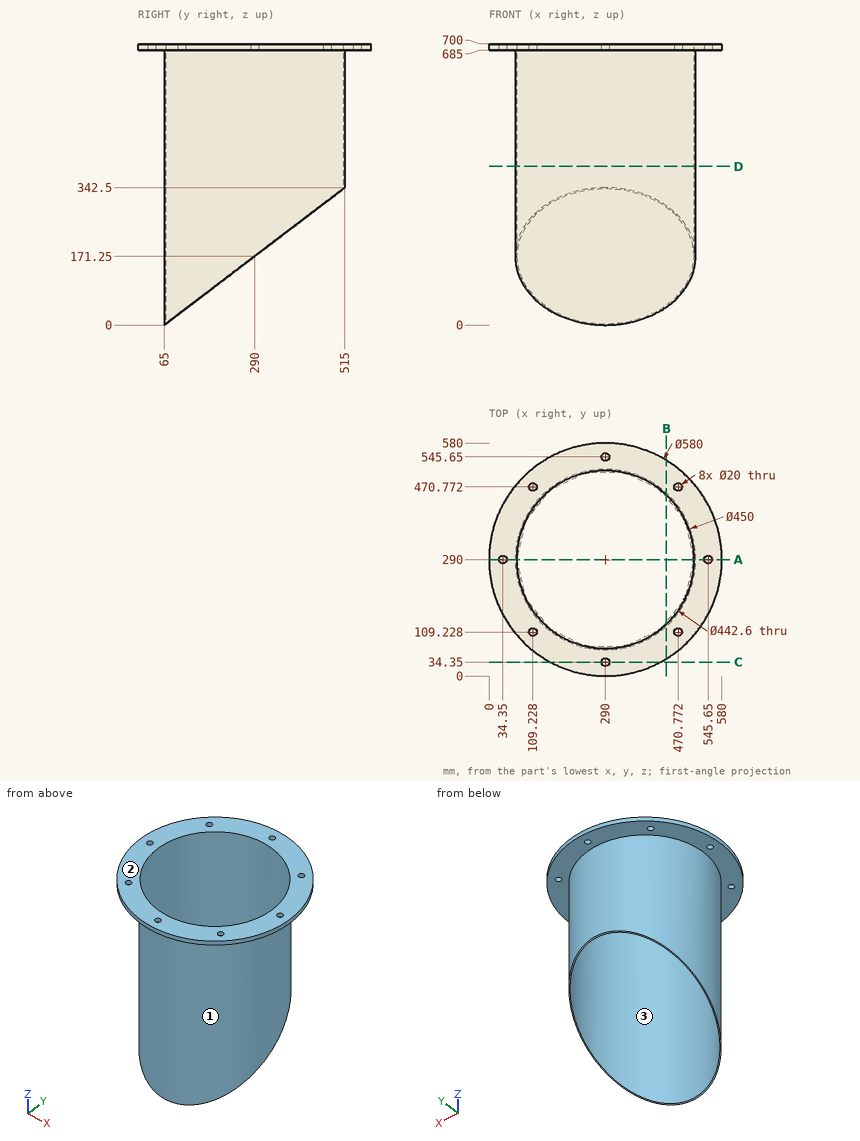
Study the drawing (mm; zero at the part's minimum x, y, z) and answer. Coordinates: 2 decimals unless noted, no trailing zeros. Write each loop counter-clockwise with the first axis right and the second up, starting at its lowest first coordinate (ties: lowest second). Pieces come first, ordered by that corner, then holes.
Q1. Each of these flat-tipped pins is pushed along its axis until it touches: pin 1 Ø23 at (x, y) = (290, 545.65) entering from +Z; pin 2 Ø6 at (y, z) = (151.5, 556) entering from +X; pin 3 Ø6 at (y, z) = (170.5, 475.5) entering from +X; pin 4 Ø4 at (x, z) = (330, 594.5) entering from -Y. Where does it stop, or does it pass through?
Q2. A cutting plane is placed at C-C, the plane y = 34.35. Give the vertices of the cut face in (x, z) (1 decimal), then the cut area to 3 significant figures.
Q3. A cutting plane is placed at B-B, the plane x = 441.5. Give the vertices of the cut face in (y, z), then the cut area to 3 significant figures.
Q4. Determine the mould class of the marked faces 1, 2 and 3 for opening direction Y: released by +Y, released by -Y, zero draft, split by the parting line, or undercut.
Q5. Find the intervals of material crossed by line 1 (Y direction, x = 290, z = 692.75); line 2 (X direction, y = 290, z = 534); line 3 (X direction, y = 341, z = 508.5), in increasing order.
Q6. A cutting plane is placed at D-D, the plane z = 395. Give the vertices of the cut face in (x, y), then the cut area to 3 significant figures.
Q7. A cutting plane is placed at A-A, the plane y = 290. Give the vertices of the cut face in (x, z), then the cut area to 3 significant figures.
Findings below:
1. pin 1: stops at z = 700
1. pin 2: stops at x = 469.62
1. pin 3: stops at x = 482.49
1. pin 4: stops at y = 68.23
2. outline: (153.1, 685) - (280, 685) - (280, 700) - (153.1, 700) - close; (300, 685) - (426.9, 685) - (426.9, 700) - (300, 700) - close
2. area: 3,810 mm2
3. outline: (42.72, 685) - (123.65, 685) - (123.65, 44.64) - (128.69, 48.47) - (128.69, 700) - (42.72, 700) - close; (451.31, 294.03) - (456.35, 297.86) - (456.35, 685) - (537.28, 685) - (537.28, 700) - (451.31, 700) - close
3. area: 7,760 mm2
4. face 1: split by the parting line
4. face 2: zero draft
4. face 3: undercut
5. line 1: y = 0 to 24.35, 44.35 to 68.7, 511.3 to 535.65, 555.65 to 580
5. line 2: x = 65 to 68.7, 511.3 to 515
5. line 3: x = 70.86 to 74.66, 505.34 to 509.14
6. outline: circle Ø450 at (290, 290); hole circle Ø442.6 at (290, 290)
6. area: 5,190 mm2
7. outline: (0, 685) - (24.35, 685) - (24.35, 700) - (0, 700) - close; (44.35, 685) - (65, 685) - (65, 171.25) - (68.7, 171.25) - (68.7, 700) - (44.35, 700) - close; (511.3, 171.25) - (515, 171.25) - (515, 685) - (535.65, 685) - (535.65, 700) - (511.3, 700) - close; (555.65, 685) - (580, 685) - (580, 700) - (555.65, 700) - close
7. area: 5,260 mm2
